Autodesk Inventor part; units mm, degrees
ref_plane "YZ Plane" through (0, 0, 0) normal (1, 0, 0) x (0, 1, 0)
ref_plane "XZ Plane" through (0, 0, 0) normal (0, 1, 0) x (-1, 0, 0)
ref_plane "XY Plane" through (0, 0, 0) normal (0, 0, 1) x (1, 0, 0)
sketch "Sketch1" plane through (0, 0, 0) normal (0, 1, 0) x (-1, 0, 0)
  circle A0 centre (-35, 35) radius 2.5
  circle A1 centre (35, -35) radius 2.5
  circle A2 centre (35, 35) radius 2.5
  circle A3 centre (-35, -35) radius 2.5
  line L0 (-35, -35) -> (35, -35) construction
  circle A4 centre (0, 0) radius 20.95
  line L1 (35, -35) -> (35, 35) construction
  line L2 (-35, 35) -> (-35, -35) construction
  line L3 (35, 35) -> (-35, 35) construction
  line L4 (-35, 35) -> (35, -35) construction
  line L5 (35, 35) -> (-35, -35) construction
  line L6 (50, 50) -> (-50, 50)
  line L7 (-50, 50) -> (-50, -50)
  line L8 (-50, -50) -> (50, -50)
  line L9 (50, -50) -> (50, 50)
  line L10 (50, 50) -> (-50, -50) construction
  line L11 (-50, 50) -> (50, -50) construction
  dimension "d4" = 41.9
  dimension "d5" = 70
  dimension "d6" = 70
  dimension "d7" = 5
  dimension "d8" = 100
  dimension "d9" = 100
extrude "Extrusion1" add sketch "Sketch1" along normal blind 10
properties part number "Bearing Plate"
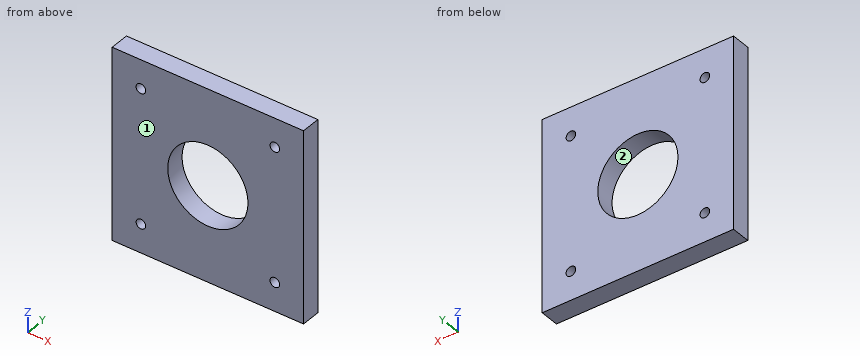
Geometry: final body of the model. Coordinates: model frame, mm. Face numbers are marked on the shaded views. Round coordinates to 2 decimals unless told otherwise and drop trailing zeros. Order: outer loops, then holes, each group sorted by start corner. A loop starts at its lowest first (then second) coordinate and runs counter-clockwise, first axis right, second up. Notation, with made-up numbers: (-28.75, -12.5) - (-6.75, -12.5) arc R21 ccw to (-6.75, 9.5) - close; hole circle Ø10 at (7.25, 69.25). An arc over 180 degrees is marked (long way). Write item = value, one per line. Start each with the question number.
Q1. Cut plane A-A on x = -35. Return the cut outline in (y, z), and give its area (3 significant figures).
Q2. Cut plane B-B on z = 0. Return the cut outline in (x, y).
Q3. Ray query, line 1 (Z direction, x = -35, y = 7.75); line 2 (Z direction, x = 0, y = 3.75); line 3 (X direction, y = 9, z = -33). Return the intervals inside material, ascending. Write a range as from..to.
Q4. Cut plane D-D on x = 0. Return the cut outline in (y, z).
Q5. Cut plane C-C on z = 35. Return the cut outline in (x, y), and give its area (3 significant figures).
Q6. Pull-direction query (Z, two-part tool) for the marked faces 1 and 2; classes: +Z half, -Z half, draft (parallel to the pull), parting line (faces both ways), or undercut.
Outcome:
q1.outline = (0, -50) - (10, -50) - (10, -37.5) - (0, -37.5) - close; (0, -32.5) - (10, -32.5) - (10, 32.5) - (0, 32.5) - close; (0, 37.5) - (10, 37.5) - (10, 50) - (0, 50) - close
q1.area = 900 mm^2
q2.outline = (-50, 0) - (-20.95, 0) - (-20.95, 10) - (-50, 10) - close; (20.95, 0) - (50, 0) - (50, 10) - (20.95, 10) - close
q3.line_1 = -50..-37.5, -32.5..32.5, 37.5..50
q3.line_2 = -50..-20.95, 20.95..50
q3.line_3 = -50..-36.5, -33.5..33.5, 36.5..50
q4.outline = (0, -50) - (10, -50) - (10, -20.95) - (0, -20.95) - close; (0, 20.95) - (10, 20.95) - (10, 50) - (0, 50) - close
q5.outline = (-50, 0) - (-37.5, 0) - (-37.5, 10) - (-50, 10) - close; (-32.5, 0) - (32.5, 0) - (32.5, 10) - (-32.5, 10) - close; (37.5, 0) - (50, 0) - (50, 10) - (37.5, 10) - close
q5.area = 900 mm^2
q6.face_1 = draft
q6.face_2 = undercut
